Autodesk Inventor part; units mm, degrees
ref_plane "YZ Plane" through (0, 0, 0) normal (1, 0, 0) x (0, 1, 0)
ref_plane "XZ Plane" through (0, 0, 0) normal (0, 1, 0) x (-1, 0, 0)
ref_plane "XY Plane" through (0, 0, 0) normal (0, 0, 1) x (1, 0, 0)
sketch "Sketch1" plane through (0, 0, 0) normal (0, 1, 0) x (-1, 0, 0)
  line L0 (82.171, 116.0061) -> (-97.829, 116.0061)
  line L1 (-97.829, 116.0061) -> (-97.829, -153.9939)
  line L2 (-97.829, -153.9939) -> (82.171, -153.9939)
  line L3 (81.171, 115.0061) -> (-96.829, 115.0061)
  line L4 (-96.829, 115.0061) -> (-96.829, -152.9939)
  line L5 (-96.829, -152.9939) -> (81.171, -152.9939)
  line L6 (81.171, 56.2728) -> (81.171, 115.0061)
  line L7 (82.171, -153.9939) -> (82.171, -93.7272)
  line L8 (82.171, 55.7393) -> (82.171, 116.0061)
  line L9 (81.171, -152.9939) -> (81.171, -94.2607)
  line L10 (-92.829, 111.0061) -> (77.171, 111.0061)
  line L11 (-92.829, 111.0061) -> (-92.829, -148.9939)
  line L12 (-92.829, -148.9939) -> (77.171, -148.9939)
  line L13 (77.171, 111.0061) -> (77.171, 58.4069)
  line L14 (77.171, -96.3948) -> (77.171, -148.9939)
  line L15 (67.171, 133.2815) -> (-82.829, 133.2815)
  line L16 (-82.829, 133.2815) -> (-82.829, 85.6394)
  line L17 (-82.829, 85.6394) -> (67.171, 85.6394)
  line L18 (67.171, 85.6394) -> (67.171, 133.2815)
  line L19 (91.8793, 101.0061) -> (59.7353, 101.0061)
  line L20 (59.7353, 101.0061) -> (59.7353, 70.7393)
  line L21 (59.7353, 70.7393) -> (91.8793, 70.7393)
  line L22 (91.8793, 70.7393) -> (91.8793, 101.0061)
  line L23 (-88.3298, 101.0061) -> (-103.1355, 101.0061)
  line L24 (-103.1355, 101.0061) -> (-103.1355, -3.9939)
  line L25 (-103.1355, -3.9939) -> (-88.3298, -3.9939)
  line L26 (-88.3298, -3.9939) -> (-88.3298, 101.0061)
  line L27 (67.171, -171.2694) -> (-82.829, -171.2694)
  line L28 (-82.829, -171.2694) -> (-82.829, -123.6273)
  line L29 (-82.829, -123.6273) -> (67.171, -123.6273)
  line L30 (67.171, -123.6273) -> (67.171, -171.2694)
  line L31 (91.8793, -138.9939) -> (59.7353, -138.9939)
  line L32 (59.7353, -138.9939) -> (59.7353, -108.7272)
  line L33 (59.7353, -108.7272) -> (91.8793, -108.7272)
  line L34 (91.8793, -108.7272) -> (91.8793, -138.9939)
  line L35 (-88.3298, -138.9939) -> (-103.1355, -138.9939)
  line L36 (-103.1355, -138.9939) -> (-103.1355, -33.9939)
  line L37 (-103.1355, -33.9939) -> (-88.3298, -33.9939)
  line L38 (-88.3298, -33.9939) -> (-88.3298, -138.9939)
  line L39 (82.171, 55.7393) -> (171.671, -4.2607)
  line L40 (82.171, -93.7272) -> (171.671, -33.7272)
  line L41 (171.671, -4.2607) -> (171.671, -33.7272)
  line L42 (90.3045, 40.9341) -> (157.1017, -3.8462)
  line L43 (107.5303, 66.6293) -> (174.3275, 21.8491)
  line L44 (107.5303, 66.6293) -> (90.3045, 40.9341)
  line L45 (174.3275, 21.8491) -> (157.1017, -3.8462)
  line L46 (174.3275, -59.837) -> (157.1017, -34.1417)
  line L47 (107.5303, -104.6172) -> (174.3275, -59.837)
  line L48 (90.3045, -78.922) -> (157.1017, -34.1417)
  line L49 (107.5303, -104.6172) -> (90.3045, -78.922)
  line L50 (170.671, -4.7942) -> (170.671, -33.1937)
  line L51 (166.671, -6.9284) -> (166.671, -31.0595)
  line L52 (166.671, -6.9284) -> (77.171, 53.0716)
  line L53 (81.171, 56.2728) -> (81.171, 55.2058)
  line L54 (77.171, 58.4069) -> (77.171, 53.0716)
  line L55 (170.671, -4.7942) -> (81.171, 55.2058)
  line L56 (35.7741, 85.6394) -> (35.6306, 85.7356)
  line L57 (166.671, -31.0595) -> (77.171, -91.0595)
  line L58 (81.171, -94.2607) -> (81.171, -93.1937)
  line L59 (77.171, -96.3948) -> (77.171, -91.0595)
  line L60 (170.671, -33.1937) -> (81.171, -93.1937)
  dimension "d0" = 270
  dimension "d3" = 1
  dimension "d4" = 1
  dimension "d5" = 1
  dimension "d17" = 5
  dimension "d30" = 5
  dimension "d31" = 1
  dimension "d32" = 15
  dimension "d33" = 15
  dimension "d34" = 15
  dimension "d35" = 15
  dimension "d38" = 15
extrude "Extrusion1" add sketch "Sketch1" along normal blind 10 contours L8 L19 L6 L3 L18 L0 | L18 L3 L16 L0 | L8 L21 L6 L19 | L16 L3 L4 L23 L1 L0 | L8 L39 L44 L55 L53 L6 L21 | L23 L4 L25 L1 | L39 L45 L55 L44 | L25 L4 L37 L1 | L39 L41 L40 L46 L60 L50 L55 L45 | L37 L4 L35 L1 | L35 L4 L5 L28 L2 L1 | L40 L49 L60 L46 | L28 L5 L30 L2 | L40 L7 L33 L9 L58 L60 L49 | L30 L5 L9 L31 L7 L2 | L7 L31 L9 L33
extrude "Extrusion2" add sketch "Sketch1" along normal blind 1 contours L18 L10 L16 L3 | L3 L6 L19 L13 L10 L18 | L6 L21 L13 L19 | L16 L10 L11 L23 L4 L3 | L6 L53 L55 L44 L52 L54 L13 L21 | L23 L11 L25 L4 | L55 L45 L52 L44 | L25 L11 L37 L4 | L55 L50 L60 L46 L57 L51 L52 L45 | L37 L11 L35 L4 | L35 L11 L12 L28 L5 L4 | L60 L49 L57 L46 | L28 L12 L30 L5 | L60 L58 L9 L33 L14 L59 L57 L49 | L30 L12 L14 L31 L9 L5 | L9 L31 L14 L33
fillet "Fillet1" radius 1 8 edges at (-81.171, 1, -123.0938) (7.829, 1, -152.9939) (-81.171, 1, 85.1059) (7.829, 1, 115.0061) (96.829, 1, -18.9939) (-125.921, 1, -63.1937) (-170.671, 1, -18.9939) (-125.921, 1, 25.2058)
extrude "Extrusion5" cut sketch "Sketch1" along normal blind 7.5 contours L18 L3 L16 L0 | L0 L16 L15 L18 | L19 L22 L21 L8 | L8 L21 L6 L19 | L18 L10 L16 L3 | L6 L21 L13 L19 | L18 L19 L20 L17 L16 L10 | L13 L21 L20 L17 L18 L19 | L23 L4 L25 L1 | L1 L25 L24 L23 | L18 L17 L20 L19 | L44 L43 L45 L39 | L39 L45 L55 L44 | L23 L11 L25 L4 | L55 L45 L52 L44 | L37 L4 L35 L1 | L1 L35 L36 L37 | L23 L26 L25 L11 | L52 L45 L42 L44 | L37 L11 L35 L4 | L37 L38 L35 L11 | L46 L47 L49 L40 | L40 L49 L60 L46 | L28 L5 L30 L2 | L2 L30 L27 L28 | L60 L49 L57 L46 | L28 L12 L30 L5 | L57 L49 L48 L46 | L28 L29 L32 L31 L30 L12 | L33 L34 L31 L7 | L7 L31 L9 L33 | L9 L31 L14 L33 | L31 L32 L29 L30 | L30 L29 L32 L33 L14 L31
sketch "Sketch3" plane through (0, 10, 0) normal (0, 1, 0) x (1, 0, 0)
  line L0 (-77.171, -53.0716) -> (-77.171, 91.0595)
  line L1 (-77.171, 91.0595) -> (-82.171, 93.7272)
  line L2 (-82.171, 93.7272) -> (-237.6798, 93.7272)
  line L3 (-237.6798, 93.7272) -> (-237.6798, -55.7393)
  line L4 (-80.171, -70.7393) -> (-80.171, -54.6722)
  line L5 (-77.171, -53.0716) -> (-82.171, -55.7393)
  line L6 (-82.171, -55.7393) -> (-237.6798, -55.7393)
  line L7 (-77.171, 18.9939) -> (139.9462, 18.9939)
  line L8 (139.9462, 18.9939) -> (139.9462, 278.7318)
  line L9 (139.9462, 278.7318) -> (-77.171, 278.7318)
  line L10 (-126.7833, 93.7272) -> (-77.171, 278.7318)
  point P0 (0, 0)
  point P1 (-81.171, -55.2058)
extrude "Extrusion9" cut sketch "Sketch3" against normal blind 100 contours L0 L1 L2 L10 L9 L8 L7 keep common part
sketch "Sketch6" plane through (96.829, 10, -18.9939) normal (0, 0, 1) x (1, 0, 0)
  line L0 (1, -10) -> (-4, -10)
  line L1 (-4, -10) -> (-4, -2.5)
  line L2 (-4, -2.5) -> (1, -2.5)
  line L3 (1, -2.5) -> (1, -10)
  point P0 (-96.829, -10)
  dimension "d68" = 7.5
  dimension "d69" = 5
extrude "Extrusion10" add sketch "Sketch6" against normal blind 1
sketch "Sketch7" plane through (-82.171, 0, -93.7272) normal (-0.4707228, 0, 0.8822811) x (0.8822811, 0, 0.4707228)
  line L0 (117.2074, 7.5) -> (-15.1347, 7.5)
  line L1 (0, 0) -> (5.6671, 0)
  line L2 (5.6671, 0) -> (5.6671, 7.5)
  line L3 (5.6671, 7.5) -> (0, 7.5)
  line L4 (0, 7.5) -> (0, 0)
  point P0 (116.6174, 0)
extrude "Extrusion11" add sketch "Sketch7" against normal blind 1
properties part number "male"
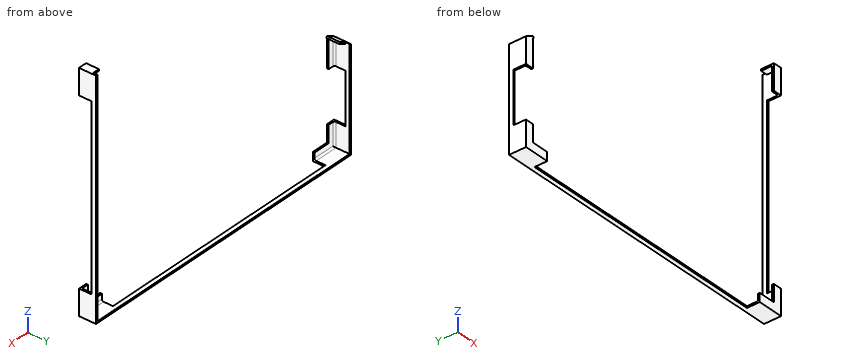
Could you check a few things on this model? Use its own coordinates, in mm. Give positions to 0.01 mm unless a question says otherwise; leave off trailing zeros. Loops run counter-clockwise (first coordinate to the right, second up) from the corner with the lowest first, then second, coordinate; pieces in that order, holes last. Notation, with made-up numbers: (-6.75, -14.5) -> (-1.75, -14.5) arc R14 ccw to (-1.75, -0.5) -> close; hole circle Ø9 at (89, 76). An arc over 180 degrees is marked (long way). Answer as CSV lines item,"result". Start each with the question number.
(1) I need wall thicknesses on probe 1 along X at (y, z) = (9.5, -96); probe 2 along X at (y, z) = (9.75, -73.5); probe 3 along Z at (x, y) = (75.5, 8.5). Which ranges of each line are inside material? Lowest first, please.
(2) If we section it at C-C on y = 5.5: Write out the boundary of the cut face in (x, z), then the cut area to 3 significant figures.
(3) If we section it at D-D on z = -76.5: Write out the boundary of the cut face in (x, y).
(4) If we section it at B-B on x = -69.5: Write out the boundary of the cut face in (y, z).
(5) If we section it at A-A on z = -135.5: Write out the boundary of the cut face in (x, y), then the cut area to 3 significant figures.
(6) I'm going to push flat-ended pins straight in: pin 1 Ø3 at (y, z) = (2, -89) entering from -X; pin 2 Ø0.8 at (x, z) = (97, -98.5) entering from -Y; pin 3 Ø0.8 at (x, y) = (-73.5, 0.5) entering from +Z; pin 4 Ø6 at (x, y) = (-8, 8.5) entering from +Z. Where does each tip first touch, or does it pass through?
Computed:
1,probe 1,"x = -82.17 to -81.17, 96.83 to 97.83"
1,probe 2,"x = 96.83 to 97.83"
1,probe 3,"z = -153.99 to -152.99"
2,outline,"(-82.17, -153.99) -> (-67.17, -153.99) -> (-67.17, -152.99) -> (-81.17, -152.99) -> (-81.17, -138.99) -> (-82.17, -138.99) -> close; (-82.17, -108.73) -> (-81.17, -108.73) -> (-81.17, -94.33) -> (-76.7, -91.94) -> (-77.17, -91.06) -> (-81.17, -93.19) -> (-82.17, -93.73) -> close; (82.83, -153.99) -> (97.83, -153.99) -> (97.83, -138.99) -> (96.83, -138.99) -> (96.83, -152.99) -> (82.83, -152.99) -> close; (92.83, -19.99) -> (96.83, -19.99) -> (96.83, -33.99) -> (97.83, -33.99) -> (97.83, -18.99) -> (92.83, -18.99) -> close"
2,area,"97.1 mm2"
3,outline,"(96.83, 7.5) -> (97.83, 7.5) -> (97.83, 10) -> (96.83, 10) -> close"
4,outline,"(0, -153.99) -> (10, -153.99) -> (10, -152.99) -> (2, -152.99) arc R1 cw to (1, -151.99) -> (1, -148.99) -> (0, -148.99) -> close"
5,outline,"(-82.17, 7.5) -> (-81.17, 7.5) -> (-81.17, 10) -> (-82.17, 10) -> close; (96.83, 7.5) -> (97.83, 7.5) -> (97.83, 10) -> (96.83, 10) -> close"
5,area,"5.00 mm2"
6,pin 1,"passes through"
6,pin 2,"stops at y = 7.5"
6,pin 3,"stops at z = -148.99"
6,pin 4,"stops at z = -152.99"
